Read the model definition and answer for the solid it produces. Units are mm, in the model's axes. Face numbers are marked on the shaded views. Give positions to 0.01 mm unless a question says otherwise; leave off trailing zeros. Loops run counter-clockwise (first coordinate to the right, second up) from the corner with the lowest first, then second, coordinate; pieces in that order, holes last. Notation, with made-up numbers: M 32,66 L 38,66 A27 cw 38,101 Z; hole C 50.5,-18 d1. An arc over 180 degrees is marked long. Return JSON: item names as keys, results as strings. Group by question number.
```python
from build123d import *

# Parameters (mm, degrees)
SKETCH1_W           = 96
SKETCH1_H           = 70.5
BOSS_EXTRUDE1_DEPTH = 3
SKETCH2_W           = 96
SKETCH2_H           = 4
BOSS_EXTRUDE2_DEPTH = 43
SKETCH3_R           = 19.798989873
CUT_EXTRUDE1_DEPTH  = 128.680264724
SKETCH4_R           = 8
SKETCH4_R_2         = 3.5
CUT_EXTRUDE2_DEPTH  = 128.680264724
BOSS_EXTRUDE3_DEPTH = 8
SKETCH6_R           = 2
CUT_EXTRUDE3_DEPTH  = 4
SKETCH7_W           = 12
SKETCH7_H           = 10
BOSS_EXTRUDE4_DEPTH = 4
SKETCH8_R           = 2
CUT_EXTRUDE4_DEPTH  = 8
CHAMFER1_SIZE       = 0.8
SKETCH9_R           = 2
CUT_EXTRUDE5_DEPTH  = 8
SKETCH10_R          = 2.9
BOSS_EXTRUDE5_DEPTH = 2
SKETCH11_R          = 2
CUT_EXTRUDE6_DEPTH  = 126.965272992
CUT_EXTRUDE7_DEPTH  = 28
SKETCH13_W          = 21.46
SKETCH13_H          = 5
CUT_EXTRUDE8_DEPTH  = 127.630367606
SKETCH14_W          = 17.46
SKETCH14_H          = 2.22
CUT_EXTRUDE9_DEPTH  = 1.5
SKETCH15_R          = 1.5
CUT_EXTRUDE10_DEPTH = 127.630367606
BOSS_EXTRUDE6_START = 1
SKETCH16_R          = 2.4
SKETCH16_R_2        = 1.5
BOSS_EXTRUDE6_DEPTH = 1
FILLET1_R           = 2


with BuildPart() as part:
    # Sketch1 → Boss-Extrude1 (new body)
    with BuildSketch(Plane(origin=(0, 0, 0), x_dir=(1, 0, 0), z_dir=(0, 1, 0))):
        with Locations((48, -35.25)):
            Rectangle(SKETCH1_W, SKETCH1_H)
    extrude(amount=BOSS_EXTRUDE1_DEPTH)

    # Sketch2 → Boss-Extrude2 (add)
    with BuildSketch(Plane(origin=(0, 3, 0), x_dir=(1, 0, 0), z_dir=(0, 1, 0))):
        with Locations((48, -2)):
            Rectangle(SKETCH2_W, SKETCH2_H)
    extrude(amount=BOSS_EXTRUDE2_DEPTH)

    # Sketch3 → Cut-Extrude1 (cut, through all)
    with BuildSketch(Plane(origin=(0, 0, 0), x_dir=(-1, 0, 0), z_dir=(0, 0, -1))):
        with Locations((-70, 23)):
            Circle(SKETCH3_R)
    extrude(amount=-CUT_EXTRUDE1_DEPTH, mode=Mode.SUBTRACT)

    # Sketch4 → Cut-Extrude2 (cut, through all)
    with BuildSketch(Plane(origin=(0, 0, 0), x_dir=(-1, 0, 0), z_dir=(0, 0, -1))):
        with Locations((-33, 14)):
            Circle(SKETCH4_R)
        with Locations((-16, 30)):
            Circle(SKETCH4_R_2)
    extrude(amount=-CUT_EXTRUDE2_DEPTH, mode=Mode.SUBTRACT)

    # Sketch5 → Boss-Extrude3 (add)
    with BuildSketch(Plane.ZY):
        Polygon((61.839745962, 3), (70.5, 8), (70.5, 3), align=None)
    boss_extrude3 = extrude(amount=-BOSS_EXTRUDE3_DEPTH)

    # Sketch6 → Cut-Extrude3 (cut)
    with BuildSketch(Plane.XY.offset(70.5)):
        with Locations((4, 4)):
            Circle(SKETCH6_R)
    cut_extrude3 = extrude(amount=-CUT_EXTRUDE3_DEPTH, mode=Mode.SUBTRACT)

    # Mirror1: Boss-Extrude3, Cut-Extrude3 across plane
    add(boss_extrude3.mirror(Plane(origin=(48, 0, 0), x_dir=(0, 0, 1), z_dir=(1, 0, 0))))
    add(cut_extrude3.mirror(Plane(origin=(48, 0, 0), x_dir=(0, 0, 1), z_dir=(1, 0, 0))), mode=Mode.SUBTRACT)

    # Sketch7 → Boss-Extrude4 (add)
    with BuildSketch(Plane(origin=(0, 46, 0), x_dir=(1, 0, 0), z_dir=(0, 1, 0))):
        with Locations((6, -5)):
            Rectangle(SKETCH7_W, SKETCH7_H)
        with Locations((90, -5)):
            Rectangle(SKETCH7_W, SKETCH7_H)
    extrude(amount=-BOSS_EXTRUDE4_DEPTH)

    # Sketch8 → Cut-Extrude4 (cut)
    with BuildSketch(Plane(origin=(0, 46, 0), x_dir=(1, 0, 0), z_dir=(0, 1, 0))):
        with Locations(Location((8, -6.5, 0), (0, 0, 270))):
            Circle(SKETCH8_R)
        with Locations(Location((88, -6.5, 0), (0, 0, 270))):
            Circle(SKETCH8_R)
    extrude(amount=-CUT_EXTRUDE4_DEPTH, mode=Mode.SUBTRACT)

    # Chamfer1
    chamfer1_edges = [part.edges().sort_by_distance(p)[0] for p in [
        (0, 46, 5),
        (96, 46, 5),
        (96, 0, 35.25),
        (0, 0, 35.25),
    ]]
    chamfer(chamfer1_edges, length=CHAMFER1_SIZE)

    # Sketch9 → Cut-Extrude5 (cut)
    with BuildSketch(Plane.XZ):
        with Locations(Location((48, 16.5, 0), (0, 0, 270))):
            Circle(SKETCH9_R)
        with Locations(Location((48, 44.5, 0), (0, 0, 270))):
            Circle(SKETCH9_R)
    extrude(amount=-CUT_EXTRUDE5_DEPTH, mode=Mode.SUBTRACT)

    # Sketch10 → Boss-Extrude5 (add)
    with BuildSketch(Plane(origin=(0, 3, 0), x_dir=(1, 0, 0), z_dir=(0, 1, 0))):
        with Locations(Location((84, -67, 0), (0, 0, 270))):
            Circle(SKETCH10_R)
        with Locations(Location((46.8, -67, 0), (0, 0, 270))):
            Circle(SKETCH10_R)
        with Locations(Location((46.8, -29.8, 0), (0, 0, 270))):
            Circle(SKETCH10_R)
        with Locations(Location((84, -29.8, 0), (0, 0, 270))):
            Circle(SKETCH10_R)
    extrude(amount=BOSS_EXTRUDE5_DEPTH)

    # Sketch11 → Cut-Extrude6 (cut, through all)
    with BuildSketch(Plane(origin=(0, 5, 0), x_dir=(1, 0, 0), z_dir=(0, 1, 0))):
        with Locations(Location((46.8, -67, 0), (0, 0, 270))):
            Circle(SKETCH11_R)
        with Locations(Location((84, -67, 0), (0, 0, 270))):
            Circle(SKETCH11_R)
        with Locations(Location((84, -29.8, 0), (0, 0, 270))):
            Circle(SKETCH11_R)
        with Locations(Location((46.8, -29.8, 0), (0, 0, 270))):
            Circle(SKETCH11_R)
    extrude(amount=-CUT_EXTRUDE6_DEPTH, mode=Mode.SUBTRACT)

    # Sketch12 → Cut-Extrude7 (cut)
    with BuildSketch(Plane.XY.offset(70.5)):
        Polygon((10.8, 3), (10.8, 2.4), (10, 2.4), (10, 0.78), (27.46, 0.78), (27.46, 2.4), (26.46, 2.4), (26.46, 3), align=None)
    extrude(amount=-CUT_EXTRUDE7_DEPTH, mode=Mode.SUBTRACT)

    # Sketch13 → Cut-Extrude8 (cut, through all)
    with BuildSketch(Plane(origin=(0, 3, 0), x_dir=(1, 0, 0), z_dir=(0, 1, 0))):
        with Locations((18.73, -46)):
            Rectangle(SKETCH13_W, SKETCH13_H)
    extrude(amount=-CUT_EXTRUDE8_DEPTH, mode=Mode.SUBTRACT)

    # Sketch14 → Cut-Extrude9 (cut)
    with BuildSketch(Plane.XY.offset(43.5)):
        with Locations((18.73, 1.89)):
            Rectangle(SKETCH14_W, SKETCH14_H)
    extrude(amount=-CUT_EXTRUDE9_DEPTH, mode=Mode.SUBTRACT)

    # Sketch15 → Cut-Extrude10 (cut, through all)
    with BuildSketch(Plane(origin=(0, 3, 0), x_dir=(1, 0, 0), z_dir=(0, 1, 0))):
        with Locations(Location((91, -47.5, 0), (0, 0, 270))):
            Circle(SKETCH15_R)
        with Locations(Location((35, -47.5, 0), (0, 0, 270))):
            Circle(SKETCH15_R)
        with Locations(Location((91, -11.5, 0), (0, 0, 270))):
            Circle(SKETCH15_R)
    extrude(amount=-CUT_EXTRUDE10_DEPTH, mode=Mode.SUBTRACT)

    # Sketch16 → Boss-Extrude6 (add)
    # profile 1 of 3: a face of its own
    with BuildSketch(Plane(origin=(0, 3, 0), x_dir=(1, 0, 0), z_dir=(0, 1, 0)).offset(BOSS_EXTRUDE6_START)):
        with Locations(Location((91, -47.5, 0), (0, 0, 270))):
            Circle(SKETCH16_R)
        with Locations(Location((91, -47.5, 0), (0, 0, 270))):
            Circle(SKETCH16_R_2, mode=Mode.SUBTRACT)
    # profile 2 of 3: a face of its own
    with BuildSketch(Plane(origin=(0, 3, 0), x_dir=(1, 0, 0), z_dir=(0, 1, 0)).offset(BOSS_EXTRUDE6_START)):
        with Locations(Location((91, -11.5, 0), (0, 0, 270))):
            Circle(SKETCH16_R)
        with Locations(Location((91, -11.5, 0), (0, 0, 270))):
            Circle(SKETCH16_R_2, mode=Mode.SUBTRACT)
    # profile 3 of 3: a face of its own
    with BuildSketch(Plane(origin=(0, 3, 0), x_dir=(1, 0, 0), z_dir=(0, 1, 0)).offset(BOSS_EXTRUDE6_START)):
        with Locations(Location((35, -47.5, 0), (0, 0, 270))):
            Circle(SKETCH16_R)
        with Locations(Location((35, -47.5, 0), (0, 0, 270))):
            Circle(SKETCH16_R_2, mode=Mode.SUBTRACT)
    extrude(amount=-BOSS_EXTRUDE6_DEPTH)

    # Fillet1
    fillet1_edges = [part.edges().sort_by_distance(p)[0] for p in [
        (84, 44, 10),
        (12, 44, 10),
    ]]
    fillet(fillet1_edges, radius=FILLET1_R)


solid = part.part
```
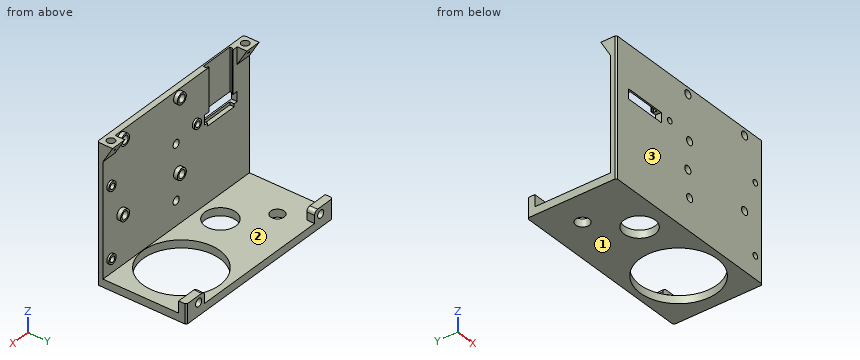
1. Find section B-B (y = 39.5). Write down the section's boundary in (x, z), and give its area (3 significant figures).
2. Flat-ended cylindrical pins translate along their axes: P1, Ø3, axis at x = 46.5, z = 67.5, coming from the +Y side; P2, Ø5, axis at x = 28, z = 12.5, coming from the +Y side; P3, Ø5, axis at x = 35, z = 47.5, coming from the +Y side. Find the tip coordinate at first contact, or state that the pin passes through.
3. Find section A-A (z = 29.8). Write down the section's boundary in (x, y), and give its area (3 significant figures).
4. The mould has two halves that part along Y. Classify the marked faces 1, 2 and 3: +Y half, -Y half, draft (parallel to the pull), parting line (faces both ways), or undercut.
5. Find section D-D (z = 16.5). Write down the section's boundary in (x, y), and give its area (3 significant figures).
6. Find section C-C (x = 35). Write down the section's boundary in (y, z).
7. Straight lines are drawn through the part: line 1 along X through (y, z) = (1, 47); line 2 along Z through (x, y) = (38, 26); line 3 along Y through (x, z) = (87, 11.5). For each, find the intervals that lie inside material, in ascending order.
Result:
{
 "1": {"outline": "M 0,0 L 59.06,0 L 59.06,4 L 0,4 Z; M 80.94,0 L 96,0 L 96,4 L 80.94,4 Z", "area": "296 mm2"},
 "2": {"P1": "stops at y = 5", "P2": "stops at y = 3", "P3": "stops at y = 4"},
 "3": {"outline": "M 0,0.8 L 0.8,0 L 44.8,0 L 44.8,5 L 43.9,5 L 43.9,3 L 0,3 Z; M 48.8,0 L 82,0 L 82,5 L 81.1,5 L 81.1,3 L 49.7,3 L 49.7,5 L 48.8,5 Z; M 86,0 L 95.2,0 L 96,0.8 L 96,3 L 86.9,3 L 86.9,5 L 86,5 Z", "area": "271 mm2"},
 "4": {"face 1": "draft", "face 2": "undercut", "face 3": "-Y half"},
 "5": {"outline": "M 0,0.8 L 0.8,0 L 46,0 L 46,3 L 0,3 Z; M 50,0 L 95.2,0 L 96,0.8 L 96,3 L 50,3 Z", "area": "275 mm2"},
 "6": {"outline": "M 0,0 L 6.25,0 L 6.25,4 L 3,4 L 3,45.1 L 4,45.1 L 4,46 L 0,46 Z; M 0,49 L 4,49 L 4,49.9 L 3,49.9 L 3,70.5 L 0,70.5 Z; M 21.75,0 L 46,0 L 46,4 L 21.75,4 Z"},
 "7": {"line 1": "x = 0 to 8, 29.46 to 33.59, 36.41 to 89.59, 92.41 to 96", "line 2": "z = 0 to 4", "line 3": "y = 0 to 3"}
}
